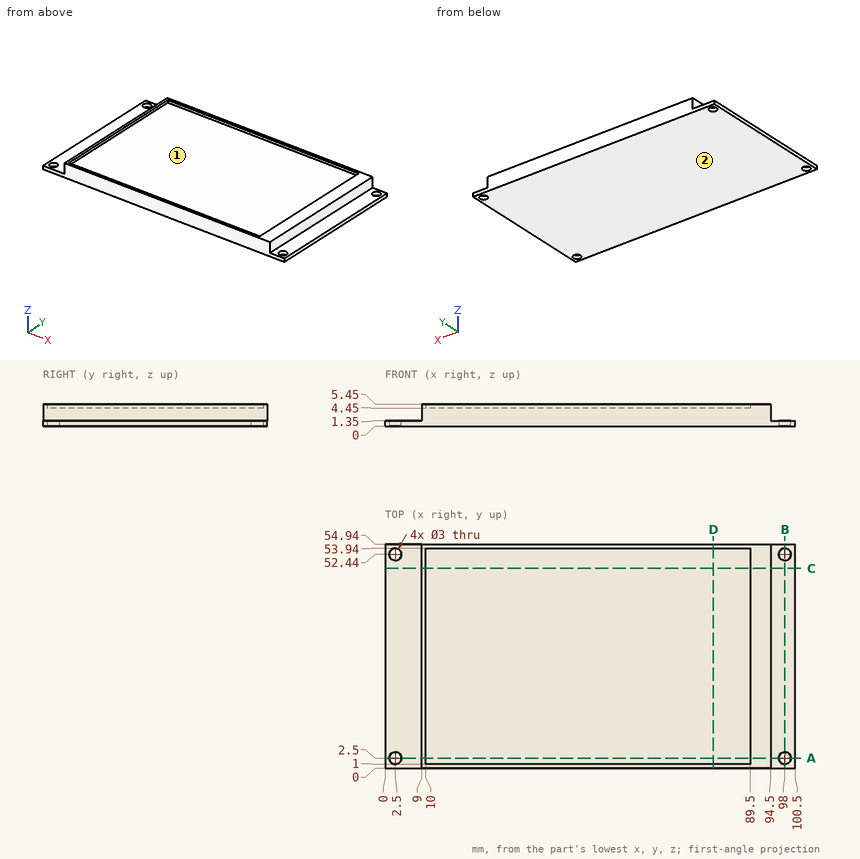
For this review, use the dimensioned drawing (mm, ordinates from the lowest corner) and the shaded views. Give positions to 0.01 mm unless a question says otherwise; leave off trailing zeros. Write each loop counter-clockwise with the first axis right and the second up, starting at its lowest first coordinate (ties: lowest second). Pieces come first, ordered by that corner, then holes. Notation, with made-up numbers: M 48.5,20 L 81.5,20 A31 cw 81.5,49 Z; hole C 7,67.5 d8. An arc over 180 degrees is marked long. Answer as a JSON object with one key per item and string values. Group by question number.
Item 1: Consider section C-C on y = 49. Write out the cut boundary in (x, z).
Item 2: For probe 1 along X at (y, z) = (52.44, 0.35); probe 2 along Y at (x, z) = (2.5, 0.5); probe 3 along Y at (x, z) = (50, 4.8), list the stretches that pass through material, from the lowest coordinate up. Write a range as [from, to].
Item 3: Consider section A-A on y = 2.5. Write out the cut boundary in (x, z).
Item 4: Consider section B-B on x = 98. Write out the cut boundary in (y, z).
Item 5: For pin 1 Ø1 at (x, y) = (74.5, 33) entering from +Z; pin 2 Ø0.5 at (y, z) = (30, 5) entering from -X; pin 3 Ø2.5 at (x, y) = (98, 52.44) entering from -Z; pin 4 Ø1.8 at (x, y) = (96, 19.5) entering from +Z, all flat-tipped, find the tip position at first contact; note any pin that passes through.
Item 6: Draft analysis for pull direction X (two halves, no side actions). For the marked faces 1 and 2, state which applies: +X half, -X half, draft (parallel to the pull), parting line (faces both ways), or undercut.
Item 7: Consider section D-D on x = 80.5. Write out the cut boundary in (y, z), plus the area to 3 significant figures.
Check result:
{
 "1": {"outline": "M 0,0 L 100.5,0 L 100.5,1.35 L 94.5,1.35 L 94.5,5.45 L 89.5,5.45 L 89.5,4.45 L 10,4.45 L 10,5.45 L 9,5.45 L 9,1.35 L 0,1.35 Z"},
 "2": {"probe 1": "x = [0, 1], [4, 96.5], [99.5, 100.5]", "probe 2": "y = [0, 1], [4, 50.94], [53.94, 54.94]", "probe 3": "y = [0, 1], [53.94, 54.94]"},
 "3": {"outline": "M 0,0 L 1,0 L 1,1.35 L 0,1.35 Z; M 4,0 L 96.5,0 L 96.5,1.35 L 94.5,1.35 L 94.5,5.45 L 89.5,5.45 L 89.5,4.45 L 10,4.45 L 10,5.45 L 9,5.45 L 9,1.35 L 4,1.35 Z; M 99.5,0 L 100.5,0 L 100.5,1.35 L 99.5,1.35 Z"},
 "4": {"outline": "M 0,0 L 1,0 L 1,1.35 L 0,1.35 Z; M 4,0 L 50.94,0 L 50.94,1.35 L 4,1.35 Z; M 53.94,0 L 54.94,0 L 54.94,1.35 L 53.94,1.35 Z"},
 "5": {"pin 1": "stops at z = 4.45", "pin 2": "stops at x = 9", "pin 3": "passes through", "pin 4": "stops at z = 1.35"},
 "6": {"face 1": "undercut", "face 2": "draft"},
 "7": {"outline": "M 0,0 L 54.94,0 L 54.94,5.45 L 53.94,5.45 L 53.94,4.45 L 1,4.45 L 1,5.45 L 0,5.45 Z", "area": "246 mm^2"}
}
